Source: CAD feature listing. Evaluate the final solid. Frame: model axes, mm. Face numbers are marked on the shaded views. A direction names the side the tool comes from. Round coordinates to 2 decimals unless told otherwise and drop trailing zeros. Order: outer loops, then holes, each group sorted by start corner. A loop starts at its lowest first (then second) coordinate and runs counter-clockwise, first axis right, second up. Notation, with made-up numbers: (18, 45.25) -> (73, 45.25) arc R8 cw to (73, 56.25) -> close; hole circle Ø11 at (-12.75, 26.25). An arc over 180 degrees is marked (long way). Answer as CSV lines item,"result".
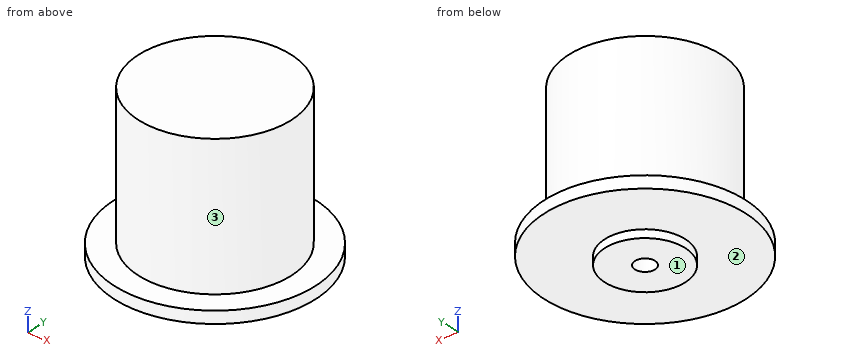
from build123d import *

# Parameters (mm, degrees)
ESQUISSE1_R             = 19
BASE_EXTRUSION_DEPTH    = 35
ESQUISSE2_R             = 25
BOSS_EXTRU_1_DEPTH      = 3
ESQUISSE3_R             = 10
BOSS_EXTRU_2_DEPTH      = 2
ESQUISSE4_R             = 2.5
ENL_V_MAT_EXTRU_1_DEPTH = 10


with BuildPart() as part:
    # Esquisse1 → Base-Extrusion (new body)
    with BuildSketch(Plane.XY):
        Circle(ESQUISSE1_R)
    extrude(amount=BASE_EXTRUSION_DEPTH)

    # Esquisse2 → Boss.-Extru.1 (add)
    with BuildSketch(Plane(origin=(0, 0, 0), x_dir=(-1, 0, 0), z_dir=(0, 0, -1))):
        Circle(ESQUISSE2_R)
    extrude(amount=BOSS_EXTRU_1_DEPTH)

    # Esquisse3 → Boss.-Extru.2 (add)
    with BuildSketch(Plane(origin=(0, 0, -3), x_dir=(-1, 0, 0), z_dir=(0, 0, -1))):
        Circle(ESQUISSE3_R)
    extrude(amount=BOSS_EXTRU_2_DEPTH)

    # Esquisse4 → Enlèv. mat.-Extru.1 (cut)
    with BuildSketch(Plane(origin=(0, 0, -5), x_dir=(-1, 0, 0), z_dir=(0, 0, -1))):
        Circle(ESQUISSE4_R)
    extrude(amount=-ENL_V_MAT_EXTRU_1_DEPTH, mode=Mode.SUBTRACT)


solid = part.part
1. Section query D-D on x = -14. Return loops of the section in (y, z), and give its area (3 significant figures).
Results below:
outline,"(-20.71, -3) -> (20.71, -3) -> (20.71, 0) -> (12.85, 0) -> (12.85, 35) -> (-12.85, 35) -> (-12.85, 0) -> (-20.71, 0) -> close"
area,"1,020 mm2"
2. Reachability of the marked faces 1, 2 and 3 from +Z, -Z, +X, -X, +Y, -Y: full face, straight path, thin tool, end or side. Return the list, or none.
Results below:
face 1,"-Z, +X, -X, +Y, -Y"
face 2,"-Z"
face 3,"+Z"
3. Line query: L1, parallel to Z at x = 10.5, y = -2.5; L2, parallel to Z at x = 13, y = 19; L3, parallel to Y at x = 0, z = 1.25. Output: solid intervals per line, ascending. Write a range as [from, to].
Results below:
L1,"[-3, 35]"
L2,"[-3, 0]"
L3,"[-19, -2.5], [2.5, 19]"
4. Section query A-A on y = 0. Return loops of the section in (x, z), and give its area (3 significant figures).
Results below:
outline,"(-25, -3) -> (-10, -3) -> (-10, -5) -> (-2.5, -5) -> (-2.5, 5) -> (2.5, 5) -> (2.5, -5) -> (10, -5) -> (10, -3) -> (25, -3) -> (25, 0) -> (19, 0) -> (19, 35) -> (-19, 35) -> (-19, 0) -> (-25, 0) -> close"
area,"1,470 mm2"
5. Section query C-C on z = 11.5. Return loops of the section in (x, y), and give its area (3 significant figures).
Results below:
outline,"circle Ø38 at (0, 0)"
area,"1,130 mm2"
6. Pin query (flat end, axial travel): pin 1 (6 mm diameter, centred on x = 7, y = -18, fed in from -Z); pin 2 (1.5 mm diameter, centred on x = 17, z = 30.5, fed in from +Y); pin 3 (5 mm diameter, centred on x = 12.5, z = 3, fed in from +Y). Return the tip coordinate at first contact, or that it passes through.
Results below:
pin 1,"z = -3"
pin 2,"y = 9.85"
pin 3,"y = 16.16"
